Could you check a few things on this model? Use its own coordinates, in mm. Face numbers are marked on the shaded views. A direction names the side the tool comes from. Give positions to 0.01 mm unless a question says otherwise; leave off trailing zeros. Loops run counter-clockwise (first coordinate to the right, second up) from the corner with the lowest first, then second, coordinate; pieces in that order, holes last. Notation, with made-up numbers: M -17.5,9.25 L 19.5,9.25 A33 cw 19.5,43.25 Z; hole C 46,83 d11. An arc over 180 degrees is marked long. Answer in a Markdown table with one row per item. Add a question column.
1. I'm going to push flat-ended pins straight in: pin 1 Ø11 at (x, y) = (75.55, 109.14) entering from -Z; pin 2 Ø10 at (x, z) = (-8.2, 79.08) entering from -Y; pin 3 Ø2 at (x, z) = (117, 29) entering from +Y. Where does each tip first touch, or does it pass through?
2. I need wall thicknesses on line 1 along Z through (x, y) = (-120, 5); line 2 along Y through (x, z) = (-120, 97); line 3 along Y through (x, z) = (-111, 100). Which ranges of each line are inside material? Lowest first, please. Write a range as from..to.
3. If we section it at C-C on y = 42.5: List the corners of the cut face in (x, z) for me, then the cut area to 3 significant figures.
4. Which directions (+Z, -Z, +X, -X, +Y, -Y) give clear straight access to the entire face, cutting with the end or side of a thin tool? Please do the marked faces 1 and 2.
5. Thinking about a two-plate mould opening in Y: for the marked faces 3, 4 and 5, which applies, released by +Y, released by -Y, zero draft, split by the parting line, or undercut?
6. If we section it at B-B on z = 37: List the corners of the cut face in (x, y) for me, then the cut area to 3 significant figures.
7. If we section it at A-A on x = 10.5: List the corners of the cut face in (y, z) for me.
```python
from build123d import *

# Parameters (mm, degrees)
SKETCH1_W           = 304.8
SKETCH1_H           = 203.2
BOSS_EXTRUDE1_DEPTH = 6.35
SKETCH2_W           = 304.8
SKETCH2_H           = 6.35
BOSS_EXTRUDE2_DEPTH = 40.64
SKETCH3_W           = 20.403275231
SKETCH3_H           = 40.64
CUT_EXTRUDE1_DEPTH  = 325.70549749
SKETCH2_2_W         = 304.8
SKETCH2_2_H         = 6.35
BOSS_EXTRUDE3_DEPTH = 203.2
SKETCH9_R           = 3.175
CUT_EXTRUDE2_DEPTH  = 10.922
SKETCH10_R          = 3.175
SKETCH10_R_2        = 3.392842108
CUT_EXTRUDE3_DEPTH  = 10.922
SKETCH11_W          = 4.440800547
SKETCH11_H          = 55.485459727
BOSS_EXTRUDE7_DEPTH = 50.8
CHAMFER1_SIZE       = 2.38
SKETCH12_W          = 5.089607789
SKETCH12_H          = 51.20183316
BOSS_EXTRUDE8_DEPTH = 50.8
CHAMFER2_SIZE       = 2.38
SKETCH13_R          = 3.175
CUT_EXTRUDE4_DEPTH  = 50.8
SKETCH14_R          = 3.175
CUT_EXTRUDE5_DEPTH  = 50.8


with BuildPart() as part:
    # Sketch1 → Boss-Extrude1 (new body)
    with BuildSketch(Plane(origin=(0, 0, 0), x_dir=(1, 0, 0), z_dir=(0, 1, 0))):
        Rectangle(SKETCH1_W, SKETCH1_H)
    extrude(amount=BOSS_EXTRUDE1_DEPTH)

    # Sketch2 → Boss-Extrude2 (add)
    with BuildSketch(Plane(origin=(0, 6.35, 0), x_dir=(1, 0, 0), z_dir=(0, 1, 0))):
        with Locations((0, -98.425)):
            Rectangle(SKETCH2_W, SKETCH2_H)
    extrude(amount=BOSS_EXTRUDE2_DEPTH)

    # Sketch3 → Cut-Extrude1 (cut, through all)
    with BuildSketch(Plane(origin=(152.4, 0, 0), x_dir=(0, 0, -1), z_dir=(1, 0, 0))):
        with Locations((-91.398362385, 26.67)):
            Rectangle(SKETCH3_W, SKETCH3_H)
        with Locations((91.398362385, 26.67)):
            Rectangle(SKETCH3_W, SKETCH3_H)
    extrude(amount=-CUT_EXTRUDE1_DEPTH, mode=Mode.SUBTRACT)

    # Sketch2_2 → Boss-Extrude3 (add)
    with BuildSketch(Plane(origin=(0, 6.35, 0), x_dir=(1, 0, 0), z_dir=(0, 1, 0))):
        with Locations((0, -98.425)):
            Rectangle(SKETCH2_2_W, SKETCH2_2_H)
    extrude(amount=BOSS_EXTRUDE3_DEPTH)

    # Sketch9 → Cut-Extrude2 (cut)
    with BuildSketch(Plane.XZ):
        with Locations(Location((-120.65, 79.078648077, 0), (0, 0, 270))):
            Circle(SKETCH9_R)
        with Locations(Location((-120.65, 18.102975355, 0), (0, 0, 270))):
            Circle(SKETCH9_R)
        with Locations(Location((-8.205, 79.078648077, 0), (0, 0, 270))):
            Circle(SKETCH9_R)
        with Locations(Location((-8.205, 18.102975355, 0), (0, 0, 270))):
            Circle(SKETCH9_R)
        with Locations(Location((75.547873201, 73.627514031, 0), (0, 0, 270))):
            Circle(SKETCH9_R)
    extrude(amount=-CUT_EXTRUDE2_DEPTH, mode=Mode.SUBTRACT)

    # Sketch10 → Cut-Extrude3 (cut)
    with BuildSketch(Plane.XY.offset(101.6)):
        with Locations((-120.65, 82.55)):
            Circle(SKETCH10_R)
        with Locations((-120.65, 21.89944615)):
            Circle(SKETCH10_R)
        with Locations((-8.205, 82.46463474)):
            Circle(SKETCH10_R)
        with Locations((-8.205, 21.81408089)):
            Circle(SKETCH10_R)
        with Locations((75.547873201, 109.138715406)):
            Circle(SKETCH10_R_2)
        with Locations((75.547873201, 20.470285647)):
            Circle(SKETCH10_R)
    extrude(amount=-CUT_EXTRUDE3_DEPTH, mode=Mode.SUBTRACT)

    # Sketch11 → Boss-Extrude7 (add)
    with BuildSketch(Plane.XY.offset(101.6)):
        with Locations((-150.179599726, 181.807270136)):
            Rectangle(SKETCH11_W, SKETCH11_H)
    extrude(amount=BOSS_EXTRUDE7_DEPTH)

    # Chamfer1
    chamfer1_edges = [part.edges().sort_by_distance(p)[0] for p in [
        (-150.179599726, 154.064540273, 101.6),
        (-147.959199453, 181.807270136, 101.6),
    ]]
    chamfer(chamfer1_edges, length=CHAMFER1_SIZE)

    # Sketch12 → Boss-Extrude8 (add)
    with BuildSketch(Plane.XZ):
        with Locations((-149.855196105, -75.99908342)):
            Rectangle(SKETCH12_W, SKETCH12_H)
    extrude(amount=BOSS_EXTRUDE8_DEPTH)

    # Chamfer2
    chamfer2_edges = [part.edges().sort_by_distance(p)[0] for p in [
        (-147.310392211, 0, -75.99908342),
        (-149.855196105, 0, -50.39816684),
    ]]
    chamfer(chamfer2_edges, length=CHAMFER2_SIZE)

    # Sketch13 → Cut-Extrude4 (cut)
    with BuildSketch(Plane(origin=(-147.310392211, 0, 0), x_dir=(0, 0, -1), z_dir=(1, 0, 0))):
        with Locations((75.99908342, -26.59)):
            Circle(SKETCH13_R)
    extrude(amount=-CUT_EXTRUDE4_DEPTH, mode=Mode.SUBTRACT)

    # Sketch14 → Cut-Extrude5 (cut)
    with BuildSketch(Plane(origin=(-147.959199453, 0, 0), x_dir=(0, 0, -1), z_dir=(1, 0, 0))):
        with Locations((-128.19, 181.807270136)):
            Circle(SKETCH14_R)
    extrude(amount=-CUT_EXTRUDE5_DEPTH, mode=Mode.SUBTRACT)


solid = part.part
```
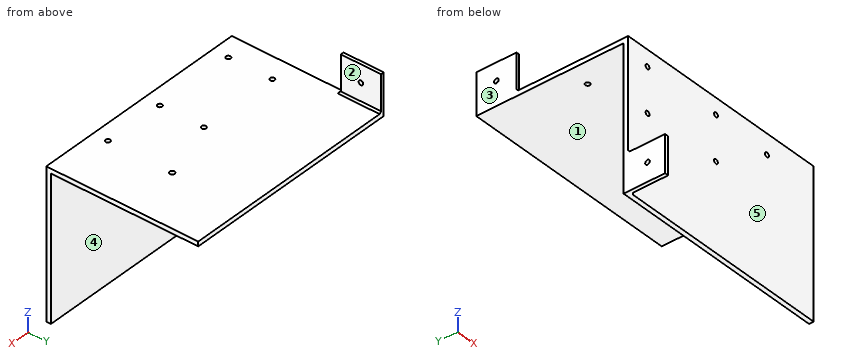
Results:
| question | item | result |
|---|---|---|
| 1 | pin 1 | z = 95.25 |
| 1 | pin 2 | y = 0 |
| 1 | pin 3 | y = 6.35 |
| 2 | line 1 | -101.6..15, 21.21..75.97, 82.19..101.6 |
| 2 | line 2 | 0..18.79, 25.01..79.44, 85.66..209.55 |
| 2 | line 3 | 0..209.55 |
| 3 | outline | M -152.4,95.25 L 152.4,95.25 L 152.4,101.6 L -152.4,101.6 Z |
| 3 | area | 1,940 mm2 |
| 4 | face 1 | -Z, +X, -X, +Y |
| 4 | face 2 | +Z, +X, +Y, -Y |
| 5 | face 3 | zero draft |
| 5 | face 4 | released by +Y |
| 5 | face 5 | released by -Y |
| 6 | outline | M -152.4,0 L 152.4,0 L 152.4,6.35 L -152.4,6.35 Z |
| 6 | area | 1,940 mm2 |
| 7 | outline | M 0,-101.6 L 6.35,-101.6 L 6.35,95.25 L 209.55,95.25 L 209.55,101.6 L 0,101.6 Z |
